```python
from build123d import *

# Parameters (mm, degrees)
SKETCH1_R           = 1.5
BOSS_EXTRUDE1_DEPTH = 1.6
SKETCH2_R           = 3.25
CUT_EXTRUDE1_DEPTH  = 1.6
FILLET1_R           = 3


with BuildPart() as part:
    # Sketch1 → Boss-Extrude1 (new body)
    with BuildSketch(Plane(origin=(0, 0, 0), x_dir=(1, 0, 0), z_dir=(0, 1, 0))):
        with BuildLine():
            ThreePointArc((168.347792712, 1300.859692621), (159.343486253, 1295.942873675), (149.343647654, 1293.65030495))
            ThreePointArc((149.343647654, 1293.65030495), (139.460555114, 1295.990018463), (130.567766275, 1300.895941835))
            ThreePointArc((130.567766275, 1300.895941835), (124.616810573, 1297.0492589), (123.648598599, 1290.029756856))
            Line((123.648598599, 1290.029756856), (131.000501903, 1282.677853551))
            ThreePointArc((131.000501903, 1282.677853551), (132.734683914, 1280.082466761), (133.343647654, 1277.020999302))
            Line((133.343647654, 1277.020999302), (133.343647654, 1272.65030495))
            Line((133.343647654, 1272.65030495), (133.343647654, 1269.65030495))
            Line((133.343647654, 1269.65030495), (133.343647654, 1240.65030495))
            Line((133.343647654, 1240.65030495), (133.343647654, 1237.65030495))
            Line((133.343647654, 1237.65030495), (133.343647654, 1233.279610599))
            ThreePointArc((133.343647654, 1233.279610599), (132.734683914, 1230.21814314), (131.000501903, 1227.622756349))
            Line((131.000501903, 1227.622756349), (123.648598599, 1220.270853045))
            ThreePointArc((123.648598599, 1220.270853045), (124.616810573, 1213.251351001), (130.567766275, 1209.404668065))
            ThreePointArc((130.567766275, 1209.404668065), (139.460555114, 1214.310591438), (149.343647654, 1216.65030495))
            ThreePointArc((149.343647654, 1216.65030495), (159.343486253, 1214.357736226), (168.347792712, 1209.44091728))
            ThreePointArc((168.347792712, 1209.44091728), (174.131892083, 1213.349250607), (175.038696709, 1220.270853045))
            Line((175.038696709, 1220.270853045), (167.686793404, 1227.622756349))
            ThreePointArc((167.686793404, 1227.622756349), (165.952611394, 1230.21814314), (165.343647654, 1233.279610599))
            Line((165.343647654, 1233.279610599), (165.343647654, 1237.65030495))
            Line((165.343647654, 1237.65030495), (165.343647654, 1240.65030495))
            Line((165.343647654, 1240.65030495), (165.343647654, 1269.65030495))
            Line((165.343647654, 1269.65030495), (165.343647654, 1272.65030495))
            Line((165.343647654, 1272.65030495), (165.343647654, 1277.020999302))
            ThreePointArc((165.343647654, 1277.020999302), (165.952611394, 1280.082466761), (167.686793404, 1282.677853551))
            Line((167.686793404, 1282.677853551), (175.038696709, 1290.029756856))
            ThreePointArc((175.038696709, 1290.029756856), (174.131892083, 1296.951359294), (168.347792712, 1300.859692621))
        make_face()
        with Locations(Location((130.843647654, 1216.65030495, 0), (0, 0, 270))):
            Circle(SKETCH1_R, mode=Mode.SUBTRACT)
        with Locations(Location((149.343647654, 1222.919184261, 0), (0, 0, 270))):
            Circle(SKETCH1_R, mode=Mode.SUBTRACT)
        with Locations(Location((167.843647654, 1216.65030495, 0), (0, 0, 270))):
            Circle(SKETCH1_R, mode=Mode.SUBTRACT)
        with Locations(Location((130.843647654, 1293.65030495, 0), (0, 0, 270))):
            Circle(SKETCH1_R, mode=Mode.SUBTRACT)
        with Locations(Location((149.343647654, 1287.38142564, 0), (0, 0, 270))):
            Circle(SKETCH1_R, mode=Mode.SUBTRACT)
        with BuildLine():
            ThreePointArc((169.343647654, 1293.65030495), (167.843647654, 1292.15030495), (166.343647654, 1293.65030495))
            ThreePointArc((166.343647654, 1293.65030495), (167.843647654, 1295.15030495), (169.343647654, 1293.65030495))
        make_face(mode=Mode.SUBTRACT)
    extrude(amount=BOSS_EXTRUDE1_DEPTH)

    # Sketch2 → Cut-Extrude1 (cut)
    with BuildSketch(Plane(origin=(0, 1.6, 0), x_dir=(1, 0, 0), z_dir=(0, 1, 0))):
        with Locations((134.093647654, 1239.90030495)):
            Circle(SKETCH2_R)
        with Locations((164.593647654, 1239.90030495)):
            Circle(SKETCH2_R)
        with Locations((164.593647654, 1270.40030495)):
            Circle(SKETCH2_R)
        with Locations((134.093647654, 1270.40030495)):
            Circle(SKETCH2_R)
    extrude(amount=-CUT_EXTRUDE1_DEPTH, mode=Mode.SUBTRACT)

    # Fillet1
    fillet1_edges = [part.edges().sort_by_distance(p)[0] for p in [
        (133.343647654, 0.8, -1243.062582611),
        (133.343647654, 0.8, -1236.73802729),
        (133.343647654, 0.8, -1273.562582611),
        (133.343647654, 0.8, -1267.23802729),
        (165.343647654, 0.8, -1267.23802729),
        (165.343647654, 0.8, -1273.562582611),
        (165.343647654, 0.8, -1236.73802729),
        (165.343647654, 0.8, -1243.062582611),
    ]]
    fillet(fillet1_edges, radius=FILLET1_R)


solid = part.part
```
Part model, mm, in its own coordinate system. A direction names the side the tool comes from. Give positions to 0.01 mm unless a question says otherwise; leave off trailing zeros. Order: outer loops, then holes, each group sorted by start corner. A loop starts at its lowest first (then second) coordinate and runs counter-clockwise, first axis right, second up. Notation, with made-up numbers: (52, 59) - (111, 59) arc R14 cw to (111, 79) - close; hole circle Ø1 at (-0.75, 52). An arc over 180 degrees is marked (long way). Use one line per item in the form item = value.
Item 1: Slice it at C-C on x = 143.5. Give the cut face in (y, z), and give its area (3 significant figures).
Solution:
outline = (0, -1294.69) - (1.6, -1294.69) - (1.6, -1215.61) - (0, -1215.61) - close
area = 127 mm2
Item 2: Probe probe 1 along Z at (x, y) = (148.5, 1.25); probe 2 along Z at (x, y) = (130.5, 1.1); probe 3 along X at (y, z) = (1.1, -1293.5). List the from-to ranges inside material, lowest first. Write a range as from..to.
Solution:
probe_1 = -1293.74..-1288.62, -1286.14..-1224.16, -1221.68..-1216.56
probe_2 = -1300.89..-1295.11, -1292.19..-1283.18, -1227.12..-1218.11, -1215.19..-1209.41
probe_3 = 123.35..129.35, 132.34..166.35, 169.34..175.34
Item 3: Which spindle directions (+Z, -Z, +X, -X, +Y, -Y) get a long thin tool onto all of the face, cutting with end or side? Do faces 4 (the face through (164.832, 0.811, -1274.555)), 5 (the face through (133.86, 0.81, -1235.75)), 6 (the face through (148.769, 0.789, -1221.534)). Say none if no direction does.
Solution:
face_4 = +X, +Y, -Y
face_5 = -X, +Y, -Y
face_6 = +Y, -Y
Item 4: Slice it at A-A on x = 172. Give the cut face in (y, z).
Solution:
outline = (0, -1299.28) - (1.6, -1299.28) - (1.6, -1286.99) - (0, -1286.99) - close; (0, -1223.31) - (1.6, -1223.31) - (1.6, -1211.02) - (0, -1211.02) - close
Item 5: Pin check, flat tips, straight feed: pin 1 Ø0.8 at (y, z) = (1, -1257.5) entering from -X; pin 2 Ø0.8 at (y, z) = (0.5, -1256.5) entering from +X. Stop position of each tip, or through.
Solution:
pin_1 = 133.34
pin_2 = 165.34
Item 6: Two-plate mould, pull along Z, no slides. Class faces 1 (the face through (159.478, 0.789, -1295.994)), 2 (the face through (133.884, 0.811, -1274.513)), 3 (the face through (139.33, 0.79, -1214.26)): released by +Z, released by -Z, zero draft, split by the parting line, or undercut.
Solution:
face_1 = released by -Z
face_2 = undercut
face_3 = released by +Z
Item 7: Slice it at B-B on z = -1279. Give the cut face in (x, y) (3 decimals), and give its area (3 significant figures).
Solution:
outline = (133.095, 0) - (165.592, 0) - (165.592, 1.6) - (133.095, 1.6) - close
area = 52.0 mm2
Item 8: Slice it at D-D on y = 0.6. Count the separate pieces of the cut face and the enclosed holes in it, and give its area (3 significant figures).
Solution:
separate_pieces = 1
enclosed_holes = 6
area = 3,010 mm2
